Job drawing, mm, ordinate dimensions from the low corner. One solid piece. A direction names the side the tool comes from. Give positions to 0.01 mm unless a question says otherwise; leave off trailing zeros. Order: outer loops, then holes, each group sorted by start corner. A loop starts at its lowest first (then second) coordinate and runs counter-clockwise, first axis right, second up. Notation, with made-up numbers: (47, 24) -> (93, 24) arc R14 cw to (93, 44) -> close; hole circle Ø2 at (-29.5, -1). An arc over 180 degrees is marked (long way). Use CSV: the item, a comma, the result in double quotes. Start each with the question number.
1. Cut at A-A on z = 4.7. List the corners of the cut face in (x, y).
2. Wall check: line 1 (X direction, y = 11, z = 4); line 2 (Y direction, x = 44, z = 1.35); line 3 (Y direction, x = 25, z = 2.9). Give the ranges that are in metal, low to high. Write a range as from..to.
3. Cut at D-D on y = 2.5. List the corners of the cut face in (x, z), then the cut area to 3 significant figures.
4. Cut at B-B on y = 11. List the corners of the cut face in (x, z).
5. 3-axis set-ups, long thin cutter, end or side, ignore diameter. For the marked faces 1, 2 and 3: which of +Z, -Z, +X, -X, +Y, -Y reach the whole face in a straight line?
6. Pull direction X, two halves, no side cores. Call the marked faces 4, 5 and 6: released by +X, released by -X, zero draft, split by the parting line, or undercut.
7. Cut at C-C on x = 25. List the corners of the cut face in (y, z), then the cut area to 3 significant figures.
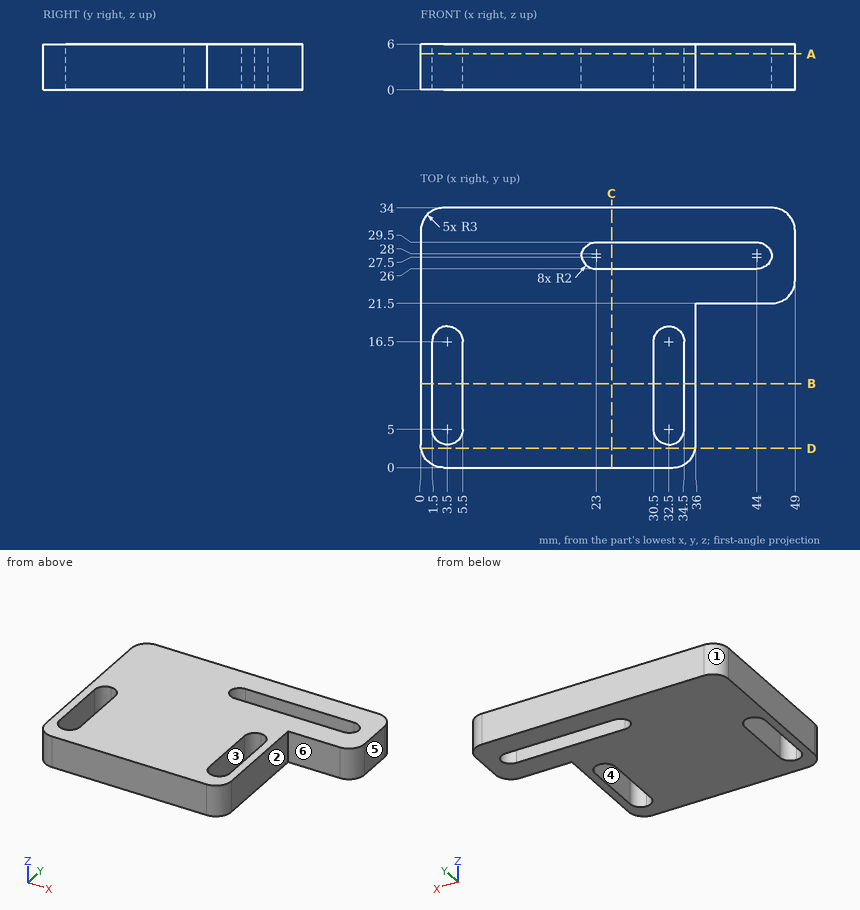
Verdict:
1,outline,"(0, 3) arc R3 ccw to (3, 0) -> (33, 0) arc R3 ccw to (36, 3) -> (36, 21.5) -> (46, 21.5) arc R3 ccw to (49, 24.5) -> (49, 31) arc R3 ccw to (46, 34) -> (3, 34) arc R3 ccw to (0, 31) -> close; hole (1.5, 5) arc R2 ccw to (5.5, 5) -> (5.5, 16.5) arc R2 ccw to (1.5, 16.5) -> close; hole (21.02, 27.75) arc R2 ccw to (23, 26) -> (44, 26) arc R2 ccw to (45.98, 27.75) arc R2 ccw to (44, 29.5) -> (23, 29.5) arc R2 ccw to start; hole (30.5, 5) arc R2 ccw to (34.5, 5) -> (34.5, 16.5) arc R2 ccw to (30.5, 16.5) -> close"
2,line 1,"0..1.5, 5.5..30.5, 34.5..36"
2,line 2,"21.5..26, 29.5..34"
2,line 3,"0..26, 29.5..34"
3,outline,"(0.04, 0) -> (35.96, 0) -> (35.96, 6) -> (0.04, 6) -> close"
3,area,"215 mm^2"
4,outline,"(0, 0) -> (1.5, 0) -> (1.5, 6) -> (0, 6) -> close; (5.5, 0) -> (30.5, 0) -> (30.5, 6) -> (5.5, 6) -> close; (34.5, 0) -> (36, 0) -> (36, 6) -> (34.5, 6) -> close"
5,face 1,"+Z, -Z, -X, +Y"
5,face 2,"+Z, -Z, +X, -Y"
5,face 3,"+Z, -Z"
6,face 4,"undercut"
6,face 5,"released by +X"
6,face 6,"zero draft"
7,outline,"(0, 0) -> (26, 0) -> (26, 6) -> (0, 6) -> close; (29.5, 0) -> (34, 0) -> (34, 6) -> (29.5, 6) -> close"
7,area,"183 mm^2"
